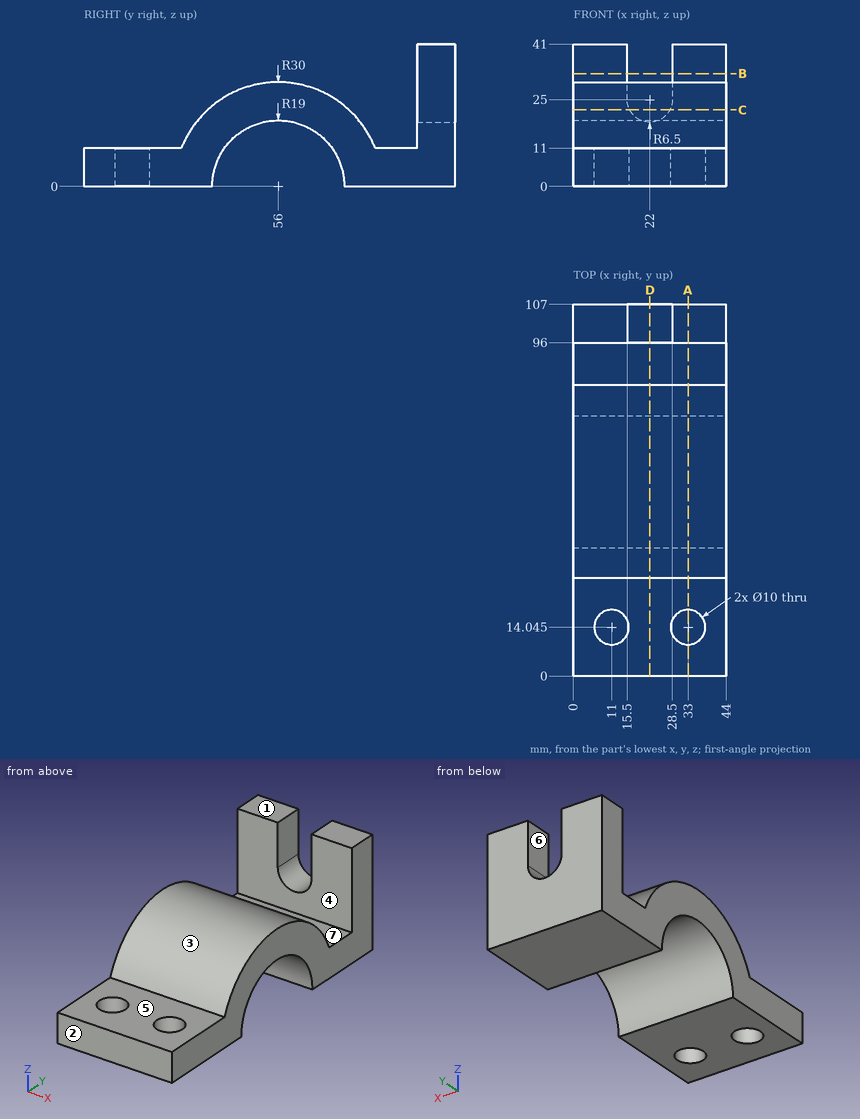
The drawing under review shows one solid part. Ordinate dimensions are in mm from its lowest x, y, z. A direction names the side the tool comes from. Coordinates: 2 decimals unless noted, no trailing zeros. Order: outer loops, then holes, each group sorted by start corner. A loop starts at its lowest first (then second) coordinate and runs counter-clockwise, first axis right, second up. Notation, with made-up numbers: M 68,6 L 105,6 A20 ccw 105,44 Z; hole C 83.25,61.25 d5. An arc over 180 degrees is marked long. One line per question, with ' | ' between items.
(1) Machinability: for the marked faces 5, 6 and 7, which of the approach directions +Z, -Z, +X, -X, +Y, -Y give a long, thin tool a straight path to every point of the face, cutting with its end or side? Answer none if there is none.
Geometry results:
face 5: +Z, +X, -X, -Y | face 6: +Z, +Y | face 7: +Z, +X, -X
(2) The part is to be moulded in two halves that separate along Y. For the marked faces 1, 2, 3 and 4, say which applies: +Y half, -Y half, draft (parallel to the pull), parting line (faces both ways), or undercut.
Geometry results:
face 1: draft | face 2: -Y half | face 3: undercut | face 4: undercut
(3) Insertion check: pin 1 (12 mm diameter, centred on x = 8.5, z = 27, fed in from -Y) (1 decimal); pin 2 (11.5 mm diameter, centred on x = 11, y = 14.04, fed in from +Z); pin 3 (10 mm diameter, centred on x = 20.5, y = 85.5, fed in from +Z); pin 4 (13 mm diameter, centred on x = 33, y = 14.04, fed in from -Z). Each pin has a flat end and moves straight along its axis. Give the tip position at first contact, or say it passes through.
Geometry results:
pin 1: stops at y = 34.6 | pin 2: stops at z = 11 | pin 3: stops at z = 17.31 | pin 4: stops at z = 0
(4) Add section D-D, the plane x = 22. Write out the cut boundary in (y, z), then the cut area to 3 significant figures.
Geometry results:
outline: M 0,0 L 37,0 A19 cw 75,0 L 107,0 L 107,18.5 L 96,18.5 L 96,11 L 83.91,11 A30 ccw 28.09,11 L 0,11 Z | area: 1,460 mm²
(5) Add section A-A, the plane x = 33. Write out the cut boundary in (y, z) (1 decimal).
Geometry results:
outline: M 0,0 L 9,0 L 9,11 L 0,11 Z; M 19,0 L 37,0 A19 cw 75,0 L 107,0 L 107,41 L 96,41 L 96,11 L 83.9,11 A30 ccw 28.1,11 L 19,11 Z
(6) Add section C-C, the plane z = 22. Write out the cut boundary in (x, y).
Geometry results:
outline: M 0,35.6 L 44,35.6 L 44,76.4 L 0,76.4 Z; M 0,96 L 16.23,96 L 16.23,107 L 0,107 Z; M 27.77,96 L 44,96 L 44,107 L 27.77,107 Z
(7) For probe 1 along Y at (x, z) = (31, 7); probe 2 along X at (y, z) = (97, 26); probe 3 along Y at (x, z) = (33, 7.25) (1 decimal), list the stretches that pass through material, from the lowest coordinate up. Write a range as from..to.
Geometry results:
probe 1: y = 0..9.46, 18.63..38.34, 73.66..107 | probe 2: x = 0..15.5, 28.5..44 | probe 3: y = 0..9, 19..38.4, 73.6..107
(8) Add section B-B, the plane z = 32.5. Write out the cut boundary in (x, y), then the cut area to 3 significant figures.
Geometry results:
outline: M 0,96 L 15.5,96 L 15.5,107 L 0,107 Z; M 28.5,96 L 44,96 L 44,107 L 28.5,107 Z | area: 341 mm²
